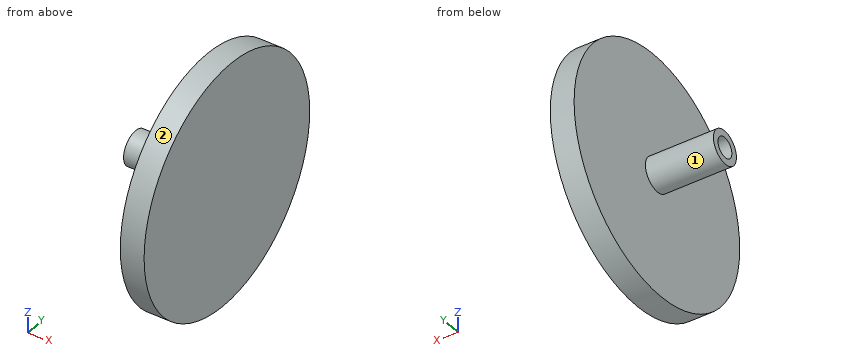
Autodesk Inventor part; units mm, degrees
ref_plane "YZ Plane" through (0, 0, 0) normal (1, 0, 0) x (0, 1, 0)
ref_plane "XZ Plane" through (0, 0, 0) normal (0, 1, 0) x (-1, 0, 0)
ref_plane "XY Plane" through (0, 0, 0) normal (0, 0, 1) x (1, 0, 0)
sketch "スケッチ1" plane through (0, 0, 0) normal (1, 0, 0) x (0, 1, 0)
  circle A0 centre (0, 0) radius 18
  dimension "d0" = 36
extrude "押し出し1" add sketch "スケッチ1" along normal blind 3.5
sketch "スケッチ2" plane through (0, 0, 0) normal (-1, 0, 0) x (0, 0, 1)
  circle A0 centre (0, 0) radius 1.5
  circle A1 centre (0, 0) radius 2.5
  dimension "d3" = 3
  dimension "d4" = 5
extrude "押し出し2" add sketch "スケッチ2" along normal blind 10
properties part number "tire" material "ゴム"
Here's how the part is built. I have some questions about the finished solid (model axes, mm). Face numbers are marked on the shaded views. A direction names the side the tool comes from. Coordinates: 2 decimals unless noted, no trailing zeros. Loops run counter-clockwise (first coordinate to the right, second up) from the corner with the lowest first, then second, coordinate; pieces in that order, holes last.
1. Imagine slicing it at D-D, the plane y = -5. Please give me the cut outline in (x, z), and give its area (3 significant figures).
2. Imagine slicing it at C-C, the plane x = -4. Please give me the cut outline in (y, z), and give its area (3 significant figures).
3. For the marked faces 1 and 2, which set-ups out of +Z, -Z, +X, -X, +Y, -Y let a thin tool reach every point of the face, with its end or its side?
4. For P1, Ø1, axis at x = 1, y = -10, coming from the -Z side; P2, Ø4, axis at x = 0.5, y = -5, coming from the +Z side, each with a flat end and sliding along its axis, tell me the tip position at first contact or that it passes through.
5. I need wall thicknesses on L1, parallel to Y at x = -3.75, z = 0; L2, parallel to X at y = 6.5, z = -8.5; L3, parallel to Z at x = -7.5, y = -2. Which ranges of each line are inside material? Lowest first, please.
6. Imagine slicing it at A-A, the plane y = 0. Please give me the cut outline in (x, z).
Taken from the geometry:
1. outline: (0, -17.29) - (3.5, -17.29) - (3.5, 17.29) - (0, 17.29) - close
1. area: 121 mm2
2. outline: circle Ø5 at (0, 0); hole circle Ø3 at (0, 0)
2. area: 12.6 mm2
3. face 1: -X
3. face 2: +X, -X
4. P1: stops at z = -15.29
4. P2: stops at z = 17.75
5. L1: y = -2.5 to -1.5, 1.5 to 2.5
5. L2: x = 0 to 3.5
5. L3: z = -1.5 to 1.5
6. outline: (-10, -2.5) - (0, -2.5) - (0, -18) - (3.5, -18) - (3.5, 18) - (0, 18) - (0, 2.5) - (-10, 2.5) - (-10, 1.5) - (0, 1.5) - (0, -1.5) - (-10, -1.5) - close
